from build123d import *

# Parameters (mm, degrees)
CUT_EXTRUDE1_DEPTH      = 20.052558883
CUT_EXTRUDE1_DEPTH_BACK = 20.052558883
SKETCH2_R               = 6.5
CUT_EXTRUDE2_DEPTH      = 18.909494689
CUT_EXTRUDE2_DEPTH_BACK = 18.909494689
SKETCH3_W               = 22.753459083
SKETCH3_H               = 0.25
SKETCH3_W_2             = 23.945473889


with BuildPart() as part:
    # Sketch1 → Revolve1 (revolve)
    with BuildSketch(Plane.XY):
        with BuildLine():
            Line((0, 11), (0, -11))
            ThreePointArc((0, -11), (11, 0), (0, 11))
        make_face()
    revolve(axis=Axis((0, 11, 0), (0, -1, 0)))

    # Sketch2 → Cut-Extrude1 (cut, two sides: drawn at the far end of the back side and taken through both)
    with BuildSketch(Plane(origin=(0, 0, 0), x_dir=(1, 0, 0), z_dir=(0, 1, 0)).offset(-CUT_EXTRUDE1_DEPTH_BACK)):
        Circle(SKETCH2_R)
    extrude(amount=CUT_EXTRUDE1_DEPTH + CUT_EXTRUDE1_DEPTH_BACK, mode=Mode.SUBTRACT)

    # Sketch3 → Cut-Extrude2 (cut, two sides: drawn at the far end of the back side and taken through both)
    with BuildSketch(Plane.XY.offset(-CUT_EXTRUDE2_DEPTH_BACK)):
        with Locations((-0.087648148, 8.749119675)):
            Rectangle(SKETCH3_W, SKETCH3_H)
        with Locations((-0.227885183, -8.749119675)):
            Rectangle(SKETCH3_W_2, SKETCH3_H)
    extrude(amount=CUT_EXTRUDE2_DEPTH + CUT_EXTRUDE2_DEPTH_BACK, mode=Mode.SUBTRACT)


solid = part.part
Can you work these out from the model? Positions are in its coordinate system, mm. Coordinates: 2 decimals unless noted, no trailing zeros. Loops run counter-clockwise (first coordinate to the right, second up) from the corner with the lowest first, then second, coordinate; pieces in that order, holes last. Notation, with made-up numbers: M -25.5,-10.5 L -19.5,-10.5 A19 ccw -19.5,18.5 Z; hole C -7,0.5 d10. An arc over 180 degrees is marked long. Return JSON: item names as keys, results as strings. Group by question number.
Item 1: If I drill on L1, parallel to Z at x = 0, y = 0; L2, parallel to X at y = -6.25, z = -0.5; L3, parallel to Z at x = 2, y = 3, over which ranges is the centre line in solid material (lowest first)? Write a range as from..to.
Item 2: Imagine slicing it at D-D (x = 8). Please give me the cut outline in (y, z), and give its area (3 significant figures).
Item 3: Imagine slicing it at C-C (y = 6.5). Please give me the cut outline in (x, z), and give its area (3 significant figures).
Item 4: Imagine slicing it at B-B (z = 0). Please give me the cut outline in (x, y).
Item 5: I'm going to push flat-ended pins straight in: pin 1 Ø2 at (x, y) = (-7.5, 5.5) entering from +Z; pin 2 Ø8 at (x, y) = (-7.5, -3) entering from +Z; pin 3 Ø10 at (x, y) = (-2.5, 2) entering from -Z. Where does each tip first touch, or does it pass through?
Item 6: Imagine slicing it at A-A (x = 0). Please give me the cut outline in (y, z).
Verdict:
{
 "1": {"L1": "z = -11..-6.5, 6.5..11", "L2": "x = -9.04..-6.48, 6.48..9.04", "L3": "z = -10.39..-6.18, 6.18..10.39"},
 "2": {"outline": "C 0,0 d15.1", "area": "179 mm^2"},
 "3": {"outline": "C 0,0 d17.75; hole C 0,0 d13", "area": "115 mm^2"},
 "4": {"outline": "M -6.83,-8.62 L -6.5,-8.62 L -6.5,8.62 L -6.83,8.62 A11 ccw Z; M 6.5,-8.62 L 6.83,-8.62 A11 ccw 6.83,8.62 L 6.5,8.62 Z"},
 "5": {"pin 1": "stops at z = 7.22", "pin 2": "stops at z = 10.22", "pin 3": "stops at z = -11"},
 "6": {"outline": "M -8.62,-6.83 A11 ccw 8.62,-6.83 L 8.62,-6.5 L -8.62,-6.5 Z; M -8.62,6.5 L 8.62,6.5 L 8.62,6.83 A11 ccw -8.62,6.83 Z"}
}
